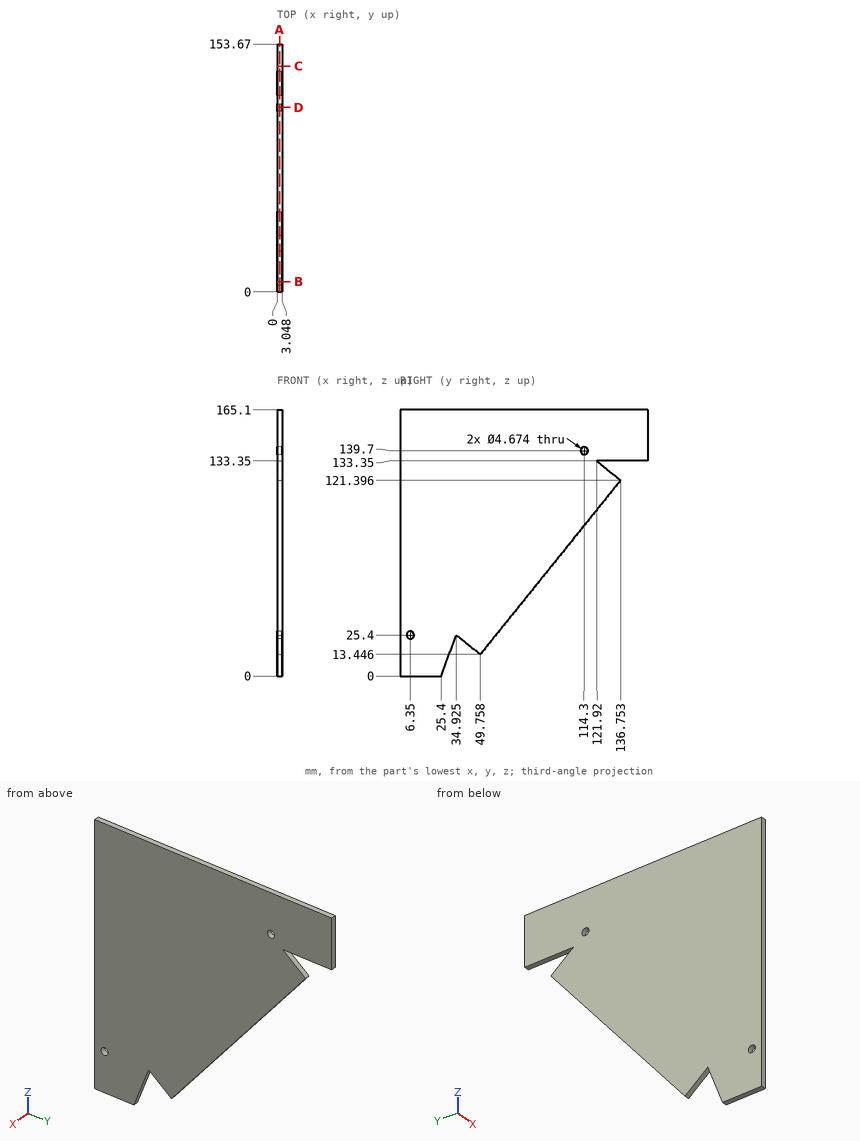
Geometry check sheet. Reference: drawing and pictorial views, mm from the part's lowest x, y, z. Give positions to 0.01 mm unless a question says otherwise; leave off trailing zeros. Loops run counter-clockwise (first coordinate to the right, second up) from the corner with the lowest first, then second, coordinate; pieces in that order, holes last. Notation, with made-up numbers: (4.25, 10) -> (26.25, 10) arc R18 cw to (26.25, 20) -> close; hole circle Ø11 at (-11.5, 13). An arc over 180 degrees is marked (long way). Answer in a Markdown table with one row per item. Add a question column.
1) Material ranges on probe 1 along Z at (x, y) = (1.4, 114.3) (1 decimal); probe 2 along Z at (x, y) = (2.4, 138.5); probe 3 along Y at (x, z) = (2.1, 15.5) (1 decimal), recorded low to high. Write a range as from..to.
2) Cross-section at C-C on y = 140. Record the boundary of the cut face in (x, z).
3) Cross-section at B-B on y = 6.35. Record the boundary of the cut face in (x, z).
4) Gauge pin test, flat end, axial feed: P1, Ø4, axis at y = 6.35, z = 25.4, coming from the -X side. Record the tip position at first contact, or that the pin passes through.
5) Cross-section at A-A on x = 1.5. State how many separate pieces and enclosed holes the cut face has, and give its area (3 significant figures).
6) Cross-section at D-D on y = 114.3. Record the boundary of the cut face in (x, z) (1 decimal).
Outcome:
| question | item | result |
|---|---|---|
| 1 | probe 1 | z = 93.5..137.4, 142..165.1 |
| 1 | probe 2 | z = 133.35..165.1 |
| 1 | probe 3 | y = 0..31.2, 47.2..51.4 |
| 2 | outline | (0, 133.35) -> (3.05, 133.35) -> (3.05, 165.1) -> (0, 165.1) -> close |
| 3 | outline | (0, 0) -> (3.05, 0) -> (3.05, 23.06) -> (0, 23.06) -> close; (0, 27.74) -> (3.05, 27.74) -> (3.05, 165.1) -> (0, 165.1) -> close |
| 4 | P1 | passes through |
| 5 | separate pieces | 1 |
| 5 | enclosed holes | 2 |
| 5 | area | 16,700 mm^2 |
| 6 | outline | (0, 93.5) -> (3, 93.5) -> (3, 137.4) -> (0, 137.4) -> close; (0, 142) -> (3, 142) -> (3, 165.1) -> (0, 165.1) -> close |
